Can you work these out from the model? Positions are in its coordinate system, mm. Face numbers are marked on the shaded views. A direction names the side the tool comes from. Coordinates: 2 decimals unless noted, no trailing zeros. Order: outer loops, then holes, each group sorted by start corner. A loop starts at its lowest first (then second) coordinate and runs counter-clockwise, first axis right, second up. Notation, with made-up numbers: (39, -26) -> (69, -26) arc R22 cw to (69, 0) -> close; hole circle Ø7 at (-27.5, -19.5). An arc over 180 degrees is marked (long way). Return JSON: item names as keys, results as strings. Group by question number.
1) If we section it at D-D, the plane y = 34.5: Please give me the cut outline in (x, z), then the cut area to 3 significant figures.
2) If I drill on probe 1 along Y at (x, z) = (15.5, 13); probe 2 along X at (y, z) = (70, 14.25); probe 3 along X at (y, z) = (51.5, 1.3), over which ranges is the centre line in solid material (lowest first)? Write a range as from..to.
3) For the marked faces 1 and 2, which set-ups out of +Z, -Z, +X, -X, +Y, -Y let a thin tool reach every point of the face, with its end or its side?
4) If we section it at B-B, the plane z = 10: Please give me the cut outline in (x, y), then the cut area to 3 significant figures.
5) Thinking about a two-plate mould opening in Y: for the marked faces 3, 4 and 5, which applies, +Y half, -Y half, draft (parallel to the pull), parting line (faces both ways), or undercut?
6) If we section it at A-A, the plane y = 51.5: Please give me the cut outline in (x, z), then the cut area to 3 significant figures.
7) For pin 1 (3 mm diameter, centred on x = 16, y = 74, fed in from +Z); pin 2 (1.5 mm diameter, centred on x = 16.35, z = 4.78, fed in from +Y); pin 3 (4 mm diameter, centred on x = 3, y = 60, fed in from +Z), each with a flat end and sliding along its axis, tell me the tip position at first contact or that it passes through.
8) If we section it at C-C, the plane x = -6: Please give me the cut outline in (y, z).
from build123d import *

# Parameters (mm, degrees)
SKETCH_1_W                  = 42
SKETCH_1_H                  = 153
EXTRUDE_1_DEPTH             = 20
SKETCH_2_W                  = 38
SKETCH_2_H                  = 149
CUT_EXTRUDE_1_DEPTH         = 17
EXTRUDE_3_DEPTH             = 17
FILLET_START                = 2
FILLET_2_DEPTH              = 18
CHAMFER_1_SIZE              = 3
CUT_EXTRUDE_3_DEPTH         = 82.812285141
SKETCH_8_R                  = 4
CUT_EXTRUDE_4_DEPTH         = 90.533513279
SKETCH_13_W                 = 27
SKETCH_13_H                 = 7.55790464
CUT_EXTRUDE_6_DEPTH         = 17
SKETCH_14_W                 = 38
SKETCH_14_H                 = 15.071373518
CUT_EXTRUDE_7_DEPTH         = 12.5
CUT_EXTRUDE_8_DEPTH         = 1
HOLE_WIZARD_M31_D           = 3.4
HOLE_WIZARD_M31_CBORE_D     = 6.5
HOLE_WIZARD_M31_CBORE_DEPTH = 3
M3X0_51_D                   = 2.5
M3X0_51_DEPTH               = 12.5
M3X0_51_TIP                 = 0.751075774
CUT_EXTRUDE_9_REACH         = 91.534
SKETCH_22_R                 = 7.5
CUT_EXTRUDE_10_REACH        = 91.534
SKETCH_23_R                 = 4


with BuildPart() as part:
    # Эскиз1 → Бобышка-Вытянуть1 (new body)
    with BuildSketch(Plane.XY):
        Rectangle(SKETCH_1_W, SKETCH_1_H)
    extrude(amount=EXTRUDE_1_DEPTH)

    # Эскиз2 → Вырез-Вытянуть1 (cut)
    with BuildSketch(Plane.XY.offset(20)):
        Rectangle(SKETCH_2_W, SKETCH_2_H)
    extrude(amount=-CUT_EXTRUDE_1_DEPTH, mode=Mode.SUBTRACT)

    # Эскиз3 → Бобышка-Вытянуть3 (add)
    with BuildSketch(Plane.XY.offset(20)):
        with BuildLine():
            Line((-19, -71), (-19, -74.5))
            Line((-19, -74.5), (-15.5, -74.5))
            ThreePointArc((-15.5, -74.5), (-13.025126266, -68.525126266), (-19, -71))
        make_face()
        with BuildLine():
            Line((19, -71), (19, -74.5))
            Line((19, -74.5), (15.5, -74.5))
            ThreePointArc((15.5, -74.5), (13.025126266, -68.525126266), (19, -71))
        make_face()
        with BuildLine():
            Line((-15.5, 55), (-19, 55))
            Line((-19, 55), (-19, 48))
            Line((-19, 48), (-15.5, 48))
            ThreePointArc((-15.5, 48), (-12, 51.5), (-15.5, 55))
        make_face()
        with BuildLine():
            Line((15.5, 55), (19, 55))
            Line((19, 55), (19, 48))
            Line((19, 48), (15.5, 48))
            ThreePointArc((15.5, 48), (12, 51.5), (15.5, 55))
        make_face()
    extrude(amount=-EXTRUDE_3_DEPTH)

    # Скругление2: read off the stored shape, not the designer's step
    # Скругление2 outline → Скругление2 (add)
    with BuildSketch(Plane.XY.offset(FILLET_START)):
        with BuildLine():
            ThreePointArc((19, 58.983314774), (17.921186974, 56.25079457), (15.266666667, 54.992213561))
            ThreePointArc((15.266666667, 54.992213561), (15.383268392, 54.998052849), (15.5, 55))
            Line((15.5, 55), (19, 55))
            Line((19, 55), (19, 58.983314774))
        make_face()
        with BuildLine():
            ThreePointArc((15.5, 48), (15.383268392, 48.001947151), (15.266666667, 48.007786439))
            ThreePointArc((15.266666667, 48.007786439), (17.921186974, 46.74920543), (19, 44.016685226))
            Line((19, 44.016685226), (19, 48))
            Line((19, 48), (15.5, 48))
        make_face()
        with BuildLine():
            ThreePointArc((15, 74.5), (17.828427125, 73.328427125), (19, 70.5))
            Line((19, 70.5), (19, 74.5))
            Line((19, 74.5), (15, 74.5))
        make_face()
        with BuildLine():
            Line((19, -71), (19, -63.516685226))
            ThreePointArc((19, -63.516685226), (17.921186974, -66.24920543), (15.266666667, -67.507786439))
            ThreePointArc((15.266666667, -67.507786439), (17.890955179, -68.443961399), (19, -71))
        make_face()
        with BuildLine():
            ThreePointArc((-19, 70.5), (-17.828427125, 73.328427125), (-15, 74.5))
            Line((-15, 74.5), (-19, 74.5))
            Line((-19, 74.5), (-19, 70.5))
        make_face()
        with BuildLine():
            ThreePointArc((15.5, -74.5), (12.943961399, -73.390955179), (12.007786439, -70.766666667))
            ThreePointArc((12.007786439, -70.766666667), (10.74920543, -73.421186974), (8.016685226, -74.5))
            Line((8.016685226, -74.5), (15.5, -74.5))
        make_face()
        with BuildLine():
            ThreePointArc((-15.266666667, 54.992213561), (-17.921186974, 56.25079457), (-19, 58.983314774))
            Line((-19, 58.983314774), (-19, 55))
            Line((-19, 55), (-15.5, 55))
            ThreePointArc((-15.5, 55), (-15.383268392, 54.998052849), (-15.266666667, 54.992213561))
        make_face()
        with BuildLine():
            Line((-15.5, -74.5), (-8.016685226, -74.5))
            ThreePointArc((-8.016685226, -74.5), (-10.74920543, -73.421186974), (-12.007786439, -70.766666667))
            ThreePointArc((-12.007786439, -70.766666667), (-12.943961399, -73.390955179), (-15.5, -74.5))
        make_face()
        with BuildLine():
            ThreePointArc((-19, 44.016685226), (-17.921186974, 46.74920543), (-15.266666667, 48.007786439))
            ThreePointArc((-15.266666667, 48.007786439), (-15.383268392, 48.001947151), (-15.5, 48))
            Line((-15.5, 48), (-19, 48))
            Line((-19, 48), (-19, 44.016685226))
        make_face()
        with BuildLine():
            ThreePointArc((-19, -71), (-17.890955179, -68.443961399), (-15.266666667, -67.507786439))
            ThreePointArc((-15.266666667, -67.507786439), (-17.921186974, -66.24920543), (-19, -63.516685226))
            Line((-19, -63.516685226), (-19, -71))
        make_face()
    extrude(amount=FILLET_2_DEPTH)

    # Фаска1
    chamfer_1_edges = [part.edges().sort_by_distance(p)[0] for p in [
        (-21, 0, 0),
        (21, 0, 0),
    ]]
    chamfer(chamfer_1_edges, length=CHAMFER_1_SIZE)

    # Эскиз7 → Вырез-Вытянуть3 (cut, through all)
    with BuildSketch(Plane.XY.offset(20)):
        with BuildLine():
            Line((-21, -71), (-21, -76.5))
            Line((-21, -76.5), (-15.5, -76.5))
            ThreePointArc((-15.5, -76.5), (-19.389087297, -74.889087297), (-21, -71))
        make_face()
        with BuildLine():
            Line((21, -76.5), (15.5, -76.5))
            ThreePointArc((15.5, -76.5), (19.389087297, -74.889087297), (21, -71))
            Line((21, -71), (21, -76.5))
        make_face()
    extrude(amount=-CUT_EXTRUDE_3_DEPTH, mode=Mode.SUBTRACT)

    # Эскиз8 → Вырез-Вытянуть4 (cut, through all)
    with BuildSketch(Plane.ZY.offset(21)):
        with Locations((-3, -58.5)):
            Circle(SKETCH_8_R)
        with Locations((-3, -38.5)):
            Circle(SKETCH_8_R)
        with Locations((-3, -18.5)):
            Circle(SKETCH_8_R)
        with Locations((-3, 1.5)):
            Circle(SKETCH_8_R)
        with Locations((-3, 21.5)):
            Circle(SKETCH_8_R)
        with Locations((-3, 41.5)):
            Circle(SKETCH_8_R)
        with Locations((-3, 61.5)):
            Circle(SKETCH_8_R)
    extrude(amount=-CUT_EXTRUDE_4_DEPTH, mode=Mode.SUBTRACT)

    # Эскиз13 → Вырез-Вытянуть6 (cut)
    with BuildSketch(Plane.XY.offset(20)):
        with Locations((0, 74.5)):
            Rectangle(SKETCH_13_W, SKETCH_13_H)
    extrude(amount=-CUT_EXTRUDE_6_DEPTH, mode=Mode.SUBTRACT)

    # Эскиз14 → Вырез-Вытянуть7 (cut)
    with BuildSketch(Plane.XY.offset(20)):
        with Locations((0, 76.5)):
            Rectangle(SKETCH_14_W, SKETCH_14_H)
    extrude(amount=-CUT_EXTRUDE_7_DEPTH, mode=Mode.SUBTRACT)

    # Эскиз15 → Вырез-Вытянуть8 (cut)
    with BuildSketch(Plane.XY.offset(20)):
        with BuildLine():
            Line((-20, 76.5), (20, 76.5))
            Line((20, 76.5), (20, -71))
            ThreePointArc((20, -71), (18.681980515, -74.181980515), (15.5, -75.5))
            Line((15.5, -75.5), (-15.5, -75.5))
            ThreePointArc((-15.5, -75.5), (-18.681980515, -74.181980515), (-20, -71))
            Line((-20, -71), (-20, 76.5))
        make_face()
    extrude(amount=-CUT_EXTRUDE_8_DEPTH, mode=Mode.SUBTRACT)

    # Цековка для винта с внутренним шестигранником M31 (through all)
    with Locations(Plane(origin=(0, 0, 0), x_dir=(-1, 0, 0), z_dir=(0, 0, -1))):
        with Locations((-15.5, 51.5), (15.5, 51.5), (15.5, -71), (-15.5, -71)):
            CounterBoreHole(HOLE_WIZARD_M31_D / 2, HOLE_WIZARD_M31_CBORE_D / 2, HOLE_WIZARD_M31_CBORE_DEPTH)

    # Отверстие обработанное метчиком M3x0.51
    with Locations(Plane(origin=(0, 76.5, 0), x_dir=(1, 0, 0), z_dir=(0, 1, 0))):
        with Locations((-16.349186161, -4.77912666), (16.349186161, -4.77912666)):
            Hole(M3X0_51_D / 2, depth=M3X0_51_DEPTH)
            with Locations((0, 0, -(M3X0_51_DEPTH + M3X0_51_TIP / 2))):  # 118° drill point
                Cone(0, M3X0_51_D / 2, M3X0_51_TIP, mode=Mode.SUBTRACT)

    # Эскиз22 → Вырез-Вытянуть9 (cut, up to next)
    with BuildSketch(Plane.ZY.offset(21), mode=Mode.PRIVATE) as cut_extrude_9_sk1:
        with Locations((19.5, 63.5)):
            Circle(SKETCH_22_R)
    cut_extrude_9_tool1 = extrude(cut_extrude_9_sk1.sketch, amount=-CUT_EXTRUDE_9_REACH, mode=Mode.PRIVATE) & part.part
    add(cut_extrude_9_tool1.solids().sort_by_distance((-21, 63.5, 19.5))[0], mode=Mode.SUBTRACT)

    # Эскиз23 → Вырез-Вытянуть10 (cut, up to next)
    with BuildSketch(Plane(origin=(21, 0, 0), x_dir=(0, 0, -1), z_dir=(1, 0, 0)), mode=Mode.PRIVATE) as cut_extrude_10_sk1:
        with Locations((-19.5, 67.89)):
            Circle(SKETCH_23_R)
    cut_extrude_10_tool1 = extrude(cut_extrude_10_sk1.sketch, amount=-CUT_EXTRUDE_10_REACH, mode=Mode.PRIVATE) & part.part
    add(cut_extrude_10_tool1.solids().sort_by_distance((21, 67.89, 19.5))[0], mode=Mode.SUBTRACT)


solid = part.part
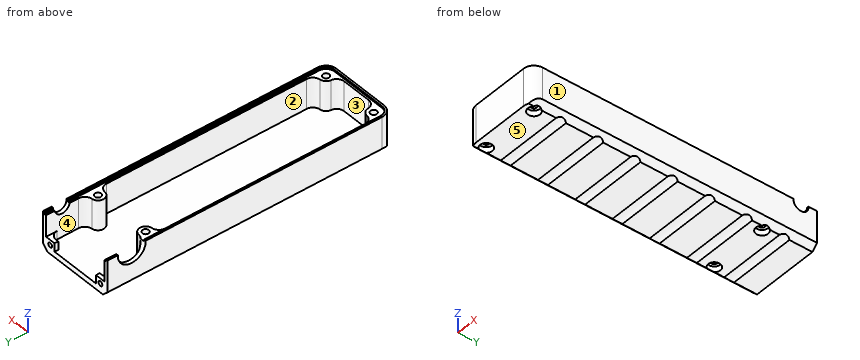
Result sheet:
{
 "1": {"outline": "(-21, 3) -> (-18, 0) -> (18, 0) -> (21, 3) -> (21, 20) -> (20, 20) -> (20, 19) -> (19, 19) -> (19, 3) -> (-19, 3) -> (-19, 19) -> (-20, 19) -> (-20, 20) -> (-21, 20) -> close", "area": "183 mm2"},
 "2": {"probe 1": "y = -76.5..-72.7, -69.3..-67.49, 47.99..49.8, 53.2..55.01", "probe 2": "x = -21..-19, 19..21", "probe 3": "x = -19.3..-18.75, -12.25..12.25, 18.75..19.3"},
 "3": {"face 1": "+Z, -Z, +X, +Y, -Y", "face 2": "+Z"},
 "4": {"outline": "(-21, -71) arc R5.5 ccw to (-15.5, -76.5) -> (15.5, -76.5) arc R5.5 ccw to (21, -71) -> (21, 76.5) -> (19, 76.5) -> (19, 58.98) arc R4 cw to (15.27, 54.99) arc R3.5 ccw to (15.27, 48.01) arc R4 cw to (19, 44.02) -> (19, -63.52) arc R4 cw to (15.27, -67.51) arc R3.5 ccw to (12.01, -70.77) arc R4 cw to (8.02, -74.5) -> (-8.02, -74.5) arc R4 cw to (-12.01, -70.77) arc R3.5 ccw to (-15.27, -67.51) arc R4 cw to (-19, -63.52) -> (-19, 44.02) arc R4 cw to (-15.27, 48.01) arc R3.5 ccw to (-15.27, 54.99) arc R4 cw to (-19, 58.98) -> (-19, 76.5) -> (-21, 76.5) -> close; hole circle Ø3.4 at (-15.5, -71); hole circle Ø3.4 at (-15.5, 51.5); hole circle Ø3.4 at (15.5, -71); hole circle Ø3.4 at (15.5, 51.5)", "area": "846 mm2"},
 "5": {"face 3": "+Y half", "face 4": "undercut", "face 5": "draft"},
 "6": {"outline": "(-21, 3) -> (-18.75, 0.75) -> (-18.75, 3) -> (-17.2, 3) -> (-17.2, 19) -> (-20, 19) -> (-20, 20) -> (-21, 20) -> close; (-13.8, 3) -> (-12.25, 3) -> (-12.25, 0) -> (12.25, 0) -> (12.25, 3) -> (13.8, 3) -> (13.8, 19) -> (12, 19) -> (12, 3) -> (-12, 3) -> (-12, 19) -> (-13.8, 19) -> close; (17.2, 3) -> (18.75, 3) -> (18.75, 0.75) -> (21, 3) -> (21, 20) -> (20, 20) -> (20, 19) -> (17.2, 19) -> close", "area": "260 mm2"},
 "7": {"pin 1": "stops at z = 7.5", "pin 2": "stops at y = 55.58", "pin 3": "stops at z = 3"},
 "8": {"outline": "(-76.5, 0) -> (-61.15, 0) arc R4 cw to (-55.85, 0) -> (-41.15, 0) arc R4 cw to (-35.85, 0) -> (-21.15, 0) arc R4 cw to (-15.85, 0) -> (-1.15, 0) arc R4 cw to (4.15, 0) -> (18.85, 0) arc R4 cw to (24.15, 0) -> (38.85, 0) arc R4 cw to (44.15, 0) -> (58.85, 0) arc R4 cw to (64.15, 0) -> (76.5, 0) -> (76.5, 3) -> (-74.5, 3) -> (-74.5, 19) -> (-75.5, 19) -> (-75.5, 20) -> (-76.5, 20) -> close"}
}
